Model file for the job. Use its own axes, mm. Coordinates: 2 decimals unless noted, no trailing zeros. Write each loop counter-clockwise with the first axis right and the second up, starting at its lowest first coordinate (ties: lowest second). Pieces come first, ordered by that corner, then holes.
Q1. Band-saw the part on B-B, the plane x = -29.5. Write the cut outline in (y, z), plus the area to 3 significant figures.
Q2. Band-saw the part on A-A, the plane z = 71. Write the cut outline in (x, y), plus the area to 3 significant figures.
Q3. Pull direction X, two halves, no side cores. Call faces 1 (the cylindrical face through (-24.977, 0.493, 1.065)), 2 (the flat face through (7, 1, 0)): released by +X, released by -X, zero draft, split by the parting line, or undercut.
Q4. Band-saw the part on C-C, the plane z = 0. Write the cut outline in (x, y).
Q5. Drill centre lines: probe 1 along X at (y, z) = (0.4, -31.5); probe 2 along Z at (x, y) = (82.5, 0.4). Where is each one in solid material? Low to high.
Q6. Band-saw the part on D-D, the plane y = 0.7. Write the cut outline in (x, z), plus the area to 3 significant figures.
from build123d import *

# Parameters (mm, degrees)
SKIZZE1_W                       = 200
SKIZZE1_H                       = 200
AUFSATZ_LINEAR_AUSTRAGEN1_DEPTH = 1


with BuildPart() as part:
    # Skizze1 → Aufsatz-Linear austragen1 (new body)
    with BuildSketch(Plane(origin=(0, 0, 0), x_dir=(1, 0, 0), z_dir=(0, 1, 0))):
        Rectangle(SKIZZE1_W, SKIZZE1_H)
        Polygon((95, 95), (-95, 95), (-95, -95), (95, -95), (95, -2.417862988), (50, -2.417862988), (50, -50), (-50, -50), (-50, 50), (50, 50), (50, 2.417862988), (95, 2.417862988), align=None, mode=Mode.SUBTRACT)
        with BuildLine():
            Line((45, 45), (-45, 45))
            Line((-45, 45), (-45, -45))
            Line((-45, -45), (45, -45))
            Line((45, -45), (45, -2.417862988))
            Line((45, -2.417862988), (24.882804074, -2.417862988))
            ThreePointArc((24.882804074, -2.417862988), (-25, 0), (24.882804074, 2.417862988))
            Line((24.882804074, 2.417862988), (45, 2.417862988))
            Line((45, 2.417862988), (45, 45))
        make_face(mode=Mode.SUBTRACT)
        with BuildLine():
            Line((0, -2.417862988), (19.853310519, -2.417862988))
            ThreePointArc((19.853310519, -2.417862988), (-20, 0), (19.853310519, 2.417862988))
            Line((19.853310519, 2.417862988), (0, 2.417862988))
            Line((0, 2.417862988), (0, -2.417862988))
        make_face(mode=Mode.SUBTRACT)
    extrude(amount=AUFSATZ_LINEAR_AUSTRAGEN1_DEPTH)


solid = part.part
Answer sheet:
1. outline: (0, -100) - (1, -100) - (1, -95) - (0, -95) - close; (0, -50) - (1, -50) - (1, -45) - (0, -45) - close; (0, 45) - (1, 45) - (1, 50) - (0, 50) - close; (0, 95) - (1, 95) - (1, 100) - (0, 100) - close
1. area: 20.0 mm2
2. outline: (-100, 0) - (-95, 0) - (-95, 1) - (-100, 1) - close; (95, 0) - (100, 0) - (100, 1) - (95, 1) - close
2. area: 10.0 mm2
3. face 1: undercut
3. face 2: zero draft
4. outline: (-100, 0) - (-95, 0) - (-95, 1) - (-100, 1) - close; (-50, 0) - (-45, 0) - (-45, 1) - (-50, 1) - close; (-25, 0) - (-20, 0) - (-20, 1) - (-25, 1) - close; (0, 0) - (100, 0) - (100, 1) - (0, 1) - close
5. probe 1: x = -100 to -95, -50 to -45, 45 to 50, 95 to 100
5. probe 2: z = -100 to -95, -2.42 to 2.42, 95 to 100
6. outline: (-100, -100) - (100, -100) - (100, 100) - (-100, 100) - close; hole (-95, -95) - (95, -95) - (95, -2.42) - (50, -2.42) - (50, -50) - (-50, -50) - (-50, 50) - (50, 50) - (50, 2.42) - (95, 2.42) - (95, 95) - (-95, 95) - close; hole (-45, -45) - (45, -45) - (45, -2.42) - (24.88, -2.42) arc R25 cw (long way) to (24.88, 2.42) - (45, 2.42) - (45, 45) - (-45, 45) - close; hole (0, -2.42) - (0, 2.42) - (19.85, 2.42) arc R20 ccw (long way) to (19.85, -2.42) - close
6. area: 6,920 mm2
